```python
from build123d import *

# Parameters (mm, degrees)
SKETCH1_W                    = 230
SKETCH1_H                    = 125.055
BASE_FLANGE1_DEPTH           = 1.3
SKETCH12_W                   = 80
SKETCH12_H                   = 15
SKETCH12_W_2                 = 15
CUT_EXTRUDE1_DEPTH           = 131.905990147
EDGE_FLANGE1_STRIP_W         = 11.2
EDGE_FLANGE1_STRIP_H         = 1.3
EDGE_FLANGE1_STRIP_CUT_DEPTH = 135
EDGE_FLANGE1_DEPTH           = 135
EDGE_FLANGE2_DEPTH           = 135
CHAMFER1_SIZE                = 10
CHAMFER1_SIZE2               = 17.320508076
CHAMFER3_SIZE                = 5
FILLET1_R                    = 5
CUT_EXTRUDE3_DEPTH           = 150.542859262
CUT_EXTRUDE3_DEPTH_BACK      = 150.542859262
SKETCH14_R                   = 2
SKETCH15_R                   = 2.65
CUT_EXTRUDE4_DEPTH           = 1.3
SKETCH16_R                   = 1.5
CUT_EXTRUDE5_DEPTH           = 1.3


# Sheet-metal steps are written as plain solids
with BuildPart() as part:
    # Sketch1 → Base-Flange1 (new body)
    with BuildSketch(Plane.XY):
        Rectangle(SKETCH1_W, SKETCH1_H)
    extrude(amount=-BASE_FLANGE1_DEPTH)

    # Sketch12 → Cut-Extrude1 (cut, through all)
    with BuildSketch(Plane.XY):
        with Locations((75, 55.0275)):
            Rectangle(SKETCH12_W, SKETCH12_H)
        with Locations((-107.5, 55.0275)):
            Rectangle(SKETCH12_W_2, SKETCH12_H)
    extrude(amount=-CUT_EXTRUDE1_DEPTH, mode=Mode.SUBTRACT)

    # Edge-Flange1 strip (across the edge) → Edge-Flange1 strip cut (cut)
    with BuildSketch(Plane(origin=(35, 62.5275, 0), x_dir=(0, -1, 0), z_dir=(-1, 0, 0))):
        with Locations((-1.3, -0.65)):
            Rectangle(EDGE_FLANGE1_STRIP_W, EDGE_FLANGE1_STRIP_H)
    extrude(amount=EDGE_FLANGE1_STRIP_CUT_DEPTH, mode=Mode.SUBTRACT)

    # Edge-Flange1 section (across the edge) → Edge-Flange1 (add)
    with BuildSketch(Plane(origin=(35, 62.5275, 0), x_dir=(0, -1, 0), z_dir=(-1, 0, 0))):
        with BuildLine():
            Line((0, 3), (0, 40.4))
            Line((0, 40.4), (1.3, 40.4))
            Line((1.3, 40.4), (1.3, 3))
            ThreePointArc((1.3, 3), (2.178679656, 0.878679656), (4.3, 0))
            Line((4.3, 0), (4.3, -1.3))
            ThreePointArc((4.3, -1.3), (1.259440841, -0.040559159), (0, 3))
        make_face()
    extrude(amount=EDGE_FLANGE1_DEPTH)

    # Edge-Flange2 section (across the edge) → Edge-Flange2 (add)
    with BuildSketch(Plane(origin=(-100, 62.5275, 50.4), x_dir=(0, 0, -1), z_dir=(1, 0, 0))):
        with BuildLine():
            Line((0, 3), (0, 18.7))
            Line((0, 18.7), (1.3, 18.7))
            Line((1.3, 18.7), (1.3, 3))
            ThreePointArc((1.3, 3), (2.178679656, 0.878679656), (4.3, 0))
            Line((4.3, 0), (10, 0))
            Line((10, 0), (10, -1.3))
            Line((10, -1.3), (4.3, -1.3))
            ThreePointArc((4.3, -1.3), (1.259440841, -0.040559159), (0, 3))
        make_face()
    extrude(amount=EDGE_FLANGE2_DEPTH)

    # Chamfer1
    chamfer1_edges = [part.edges().sort_by_distance(p)[0] for p in [
        (-100, 81.2275, 49.75),
    ]]
    chamfer1_side = [part.faces().sort_by_distance(p)[0] for p in [
        (-100, 52.8775, -0.617136938),
    ]]
    chamfer(chamfer1_edges, length=CHAMFER1_SIZE, length2=CHAMFER1_SIZE2, reference=chamfer1_side[0])

    # Chamfer3
    chamfer3_edges = [part.edges().sort_by_distance(p)[0] for p in [
        (35, 81.2275, 49.75),
    ]]
    chamfer(chamfer3_edges, length=CHAMFER3_SIZE)

    # Fillet1
    fillet1_edges = [part.edges().sort_by_distance(p)[0] for p in [
        (115, 47.5275, -0.65),
        (35, 47.5275, -0.65),
        (-115, 47.5275, -0.65),
        (-100, 47.5275, -0.65),
        (115, -62.5275, -0.65),
        (-115, -62.5275, -0.65),
    ]]
    fillet(fillet1_edges, radius=FILLET1_R)

    # Sketch14 → Cut-Extrude3 (cut, two sides: drawn at the far end of the back side and taken through both)
    with BuildSketch(Plane(origin=(0, 0, 49.1), x_dir=(-1, 0, 0), z_dir=(0, 0, -1)).offset(-CUT_EXTRUDE3_DEPTH_BACK)):
        with Locations((-21.722047565, 72.3475)):
            Circle(SKETCH14_R)
        with Locations((28.277952435, 72.3475)):
            Circle(SKETCH14_R)
        with Locations((78.277952435, 72.3475)):
            Circle(SKETCH14_R)
        with BuildLine():
            Line((-105, -49.5275), (105, -49.5275))
            ThreePointArc((105, -49.5275), (108, -52.5275), (105, -55.5275))
            Line((105, -55.5275), (-105, -55.5275))
            ThreePointArc((-105, -55.5275), (-108, -52.5275), (-105, -49.5275))
        make_face()
    extrude(amount=CUT_EXTRUDE3_DEPTH + CUT_EXTRUDE3_DEPTH_BACK, mode=Mode.SUBTRACT)

    # Sketch15 → Cut-Extrude4 (cut)
    with BuildSketch(Plane(origin=(0, 0, -1.3), x_dir=(-1, 0, 0), z_dir=(0, 0, -1))):
        with Locations((35.5, 0.4725)):
            Circle(SKETCH15_R)
        with Locations((100.5, 0.4725)):
            Circle(SKETCH15_R)
    extrude(amount=-CUT_EXTRUDE4_DEPTH, mode=Mode.SUBTRACT)

    # Sketch16 → Cut-Extrude5 (cut)
    with BuildSketch(Plane(origin=(0, 0, -1.3), x_dir=(-1, 0, 0), z_dir=(0, 0, -1))):
        with Locations((90, 33.2275)):
            Circle(SKETCH16_R)
        with Locations((-5.5, 33.2275)):
            Circle(SKETCH16_R)
        with Locations((-5.5, -11.3725)):
            Circle(SKETCH16_R)
        with Locations((90, -11.3725)):
            Circle(SKETCH16_R)
    extrude(amount=-CUT_EXTRUDE5_DEPTH, mode=Mode.SUBTRACT)


solid = part.part
```
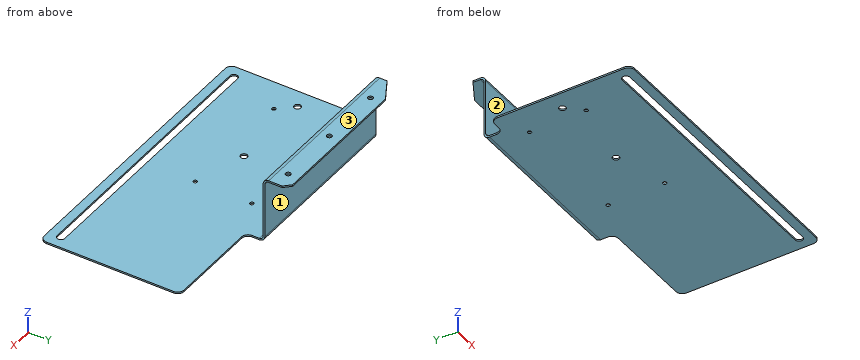
Can you work these out from the model? Positions are in its coordinate system, mm. Face numbers are marked on the shaded views. A direction names the side the tool comes from. Give positions to 0.01 mm unless a question says otherwise; leave off trailing zeros. Order: outer loops, then holes, each group sorted by start corner. A loop starts at its lowest first (then second) coordinate and runs counter-clockwise, first axis right, second up. Notation, with made-up numbers: M -19.5,-21.5 L 11.5,-21.5 A18 ccw 11.5,10.5 Z; hole C 49,76.5 d10. An arc over 180 degrees is marked long. One line per item, written item: value.
1) I want a section at D-D, the plane y = 26. List the corners of the cut face in (x, z) for me, plus the area to 3 significant figures.
Answer sheet:
outline: M -115,-1.3 L 115,-1.3 L 115,0 L -115,0 Z
area: 299 mm^2
2) Please list where these lines run through material, in increasing order: line 1 along Y through (x, z) = (-100.5, -0.8); line 2 along Y through (x, z) = (-90, -0.3); line 3 along Y through (x, z) = (-90, -0.55).
Answer sheet:
line 1: y = -62.53 to -55.53, -49.53 to -2.18, 3.12 to 50.35
line 2: y = -62.53 to -55.53, -49.53 to -12.87, -9.87 to 31.73, 34.73 to 60.98
line 3: y = -62.53 to -55.53, -49.53 to -12.87, -9.87 to 31.73, 34.73 to 60.65
3) On a 3-axis mill with a long thin cutter (end or side, diameter ignored), from which of +Z, -Z, +X, -X, +Y, -Y can I reach the whole of each face in a straight line? I mean the marked faces 1, 2 and 3. Say none if no direction works.
Answer sheet:
face 1: -Z, +X, -X, +Y
face 2: +Z, +X, -X, -Y
face 3: +Z, +X, -X, +Y, -Y
4) For P1, Ø3.5, axis at x = -90, y = 33.23, coming from the +Z side; P2, Ø12, axis at y = 61, z = 26.5, coming from the +X side; P3, Ø1.5, axis at x = 27, z = 17.5, coming from the -Y side, each with a flat end and sliding along its axis, tell me the tip position at first contact or that it passes through.
Answer sheet:
P1: stops at z = 0
P2: stops at x = 35
P3: stops at y = 61.23
5) I want a section at B-B, the plane x = 101.5. List the corners of the cut face in (y, z) for me.
Answer sheet:
outline: M -62.53,-1.3 L -55.53,-1.3 L -55.53,0 L -62.53,0 Z; M -49.53,-1.3 L 47.53,-1.3 L 47.53,0 L -49.53,0 Z
6) I want a section at A-A, the plane x = -35.5. List the corners of the cut face in (y, z) for me, plus the area to 3 significant figures.
Answer sheet:
outline: M -62.53,-1.3 L -55.53,-1.3 L -55.53,0 L -62.53,0 Z; M -49.53,-1.3 L -2.18,-1.3 L -2.18,0 L -49.53,0 Z; M 3.12,-1.3 L 58.23,-1.3 A4.3 ccw 62.53,3 L 62.53,46.1 A3 cw 65.53,49.1 L 81.23,49.1 L 81.23,50.4 L 65.53,50.4 A4.3 ccw 61.23,46.1 L 61.23,3 A3 cw 58.23,0 L 3.12,0 Z
area: 234 mm^2
7) I want a section at C-C, the plane z = 7. List the corners of the cut face in (x, y) for me, plus the area to 4 significant figures.
Answer sheet:
outline: M -100,61.23 L 35,61.23 L 35,62.53 L -100,62.53 Z
area: 175.5 mm^2
